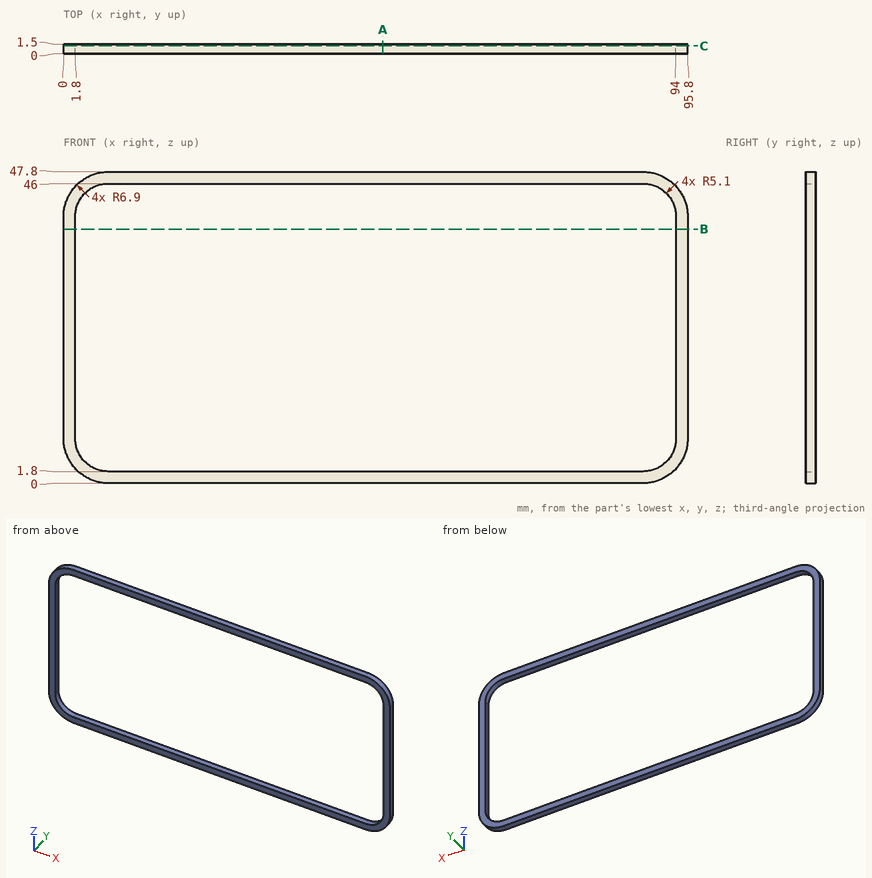
For this review, use the dimensioned drawing (mm, ordinates from the lowest corner) and the shaded views. Round coordinates to 2 decimals unless told otherwise and drop trailing zeros. Write each loop counter-clockwise with the first axis right and the second up, starting at its lowest first coordinate (ties: lowest second). Pieces come first, ordered by that corner, then holes. Notation, with made-up numbers: (63, 39.5) - (92, 39.5) arc R22 ccw to (92, 76.5) - close; hole circle Ø6 at (65, -13). An arc over 180 degrees is marked (long way). Answer as CSV lines item,"result". Start each with the question number.
(1) We need section C-C on y = 1.2. State the section outline as (x, z) points, plus the area to 3 significant figures.
(2) We need section A-A on x = 49. State the section outline as (y, z) points, plus the area to 3 significant figures.
(3) To check wall thickness, follow line 1 (Z direction, x = 35.5, y = 0.4); line 2 (X direction, y = 0.65, z = 12.5); line 3 (X direction, y = 0.95, z = 44). State the ranges of each line that lie inside material, in increasing order.
(4) We need section B-B on z = 39. State the section outline as (x, y) points.
Worked answers:
1,outline,"(0, 6.9) arc R6.9 ccw to (6.9, 0) - (88.9, 0) arc R6.9 ccw to (95.8, 6.9) - (95.8, 40.9) arc R6.9 ccw to (88.9, 47.8) - (6.9, 47.8) arc R6.9 ccw to (0, 40.9) - close; hole (1.8, 6.9) arc R5.1 ccw to (6.9, 1.8) - (88.9, 1.8) arc R5.1 ccw to (94, 6.9) - (94, 40.9) arc R5.1 ccw to (88.9, 46) - (6.9, 46) arc R5.1 ccw to (1.8, 40.9) - close"
1,area,"485 mm²"
2,outline,"(0, 0) - (1.5, 0) - (1.5, 1.8) - (0, 1.8) - close; (0, 46) - (1.5, 46) - (1.5, 47.8) - (0, 47.8) - close"
2,area,"5.40 mm²"
3,line 1,"0 to 1.8, 46 to 47.8"
3,line 2,"0 to 1.8, 94 to 95.8"
3,line 3,"0.74 to 2.85, 92.95 to 95.06"
4,outline,"(0, 0) - (1.8, 0) - (1.8, 1.5) - (0, 1.5) - close; (94, 0) - (95.8, 0) - (95.8, 1.5) - (94, 1.5) - close"
